Study the drawing (mm; zero at the part's minimum x, y, z) and answer. Coordinates: 2 decimals unless noted, no trailing zeros. Order: outer loops, then holes, each group sorted by start corner. A loop starts at its lowest first (then second) coordinate and runs counter-clockwise, first axis right, second up. Notation, with made-up numbers: M -4,83.5 L 9,83.5 A26 cw 9,100.5 Z; hole C -9,55 d9. An arc over 180 degrees is marked long. One line per item, written item: value. Start each with the question number.
Q1. Straight lines are drawn through the part: line 1 along Z through (x, y) = (4.88, 5.5) (1 decimal); line 2 along Z through (x, y) = (28.73, 6.95); line 3 along Y through (x, z) = (31.5, 18). For each, find the intervals that lie inside material, in ascending order. Write a range as [from, to].
Q2. The part is cut by section A-A on y = 2.25. Give the vertices of the cut face in (x, z), then the cut area to 3 significant figures.
Q3. The part is cut by section D-D on x = 28.73. Give the vertices of the cut face in (y, z).
Q4. The part is cut by section B-B on x = 4.88. Give the vertices of the cut face in (y, z) (1 decimal), then the cut area to 3 significant figures.
Q5. The part is cut by section C-C on z = 23. Give the vertices of the cut face in (x, y).
Q6. Each of these flat-tipped pins is pushed along its axis until it touches: pin 1 Ø1.5 at (x, y) = (5.5, 1.5) entering from -Z; pin 2 Ø2.5 at (x, y) = (17, 1.5) entering from +Z; pin 3 Ø5 at (x, z) = (9, 13.5) entering from -Y; pin 4 Ø4 at (x, z) = (23, 24) entering from -Y. Where does it stop, or does it pass through?
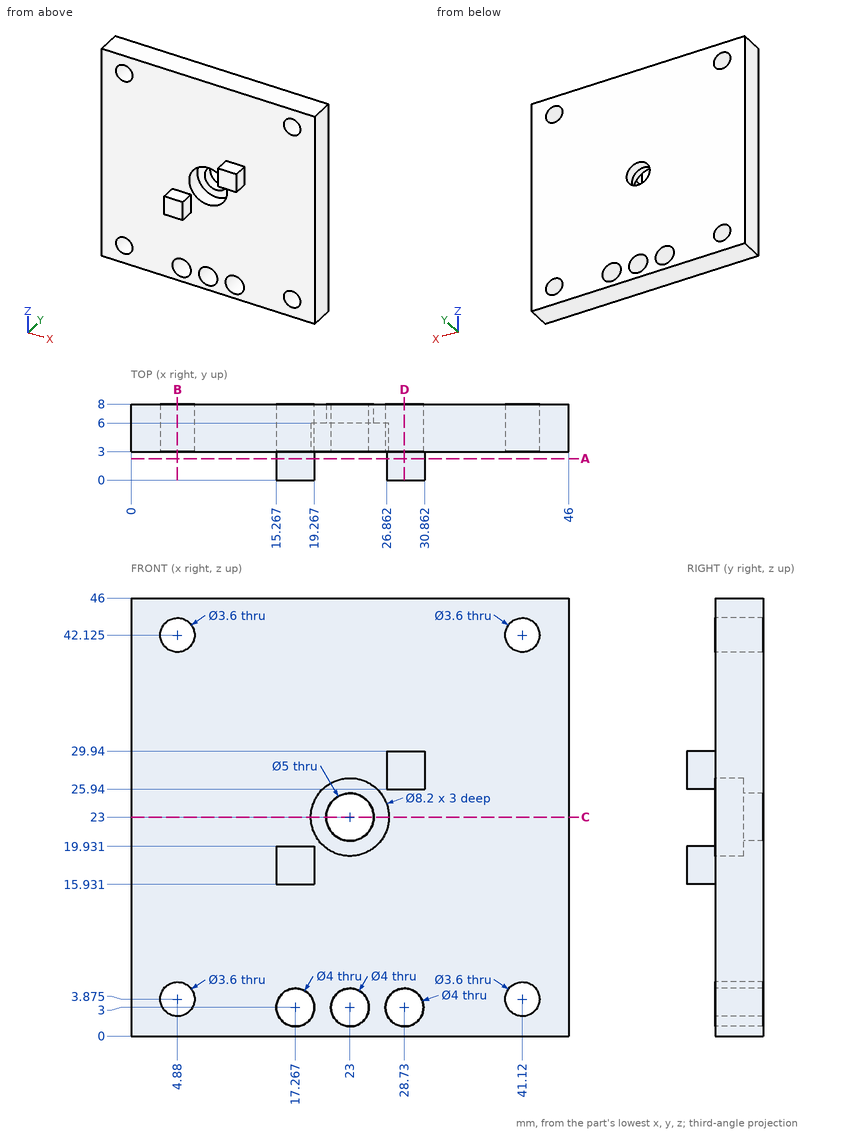
Output:
1. line 1: z = [0, 2.1], [5.7, 40.3], [43.9, 46]
1. line 2: z = [0, 1], [5, 46]
1. line 3: y = [3, 8]
2. outline: M 15.27,15.93 L 19.27,15.93 L 19.27,19.93 L 15.27,19.93 Z; M 26.86,25.94 L 30.86,25.94 L 30.86,29.94 L 26.86,29.94 Z
2. area: 32.0 mm^2
3. outline: M 0,25.94 L 3,25.94 L 3,5 L 8,5 L 8,46 L 3,46 L 3,29.94 L 0,29.94 Z; M 3,0 L 8,0 L 8,1 L 3,1 Z
4. outline: M 3,0 L 8,0 L 8,2.1 L 3,2.1 Z; M 3,5.7 L 8,5.7 L 8,40.3 L 3,40.3 Z; M 3,43.9 L 8,43.9 L 8,46 L 3,46 Z
4. area: 194 mm^2
5. outline: M 0,3 L 18.9,3 L 18.9,6 L 20.5,6 L 20.5,8 L 0,8 Z; M 25.5,6 L 27.1,6 L 27.1,3 L 46,3 L 46,8 L 25.5,8 Z
6. pin 1: passes through
6. pin 2: stops at z = 19.93
6. pin 3: stops at y = 3
6. pin 4: stops at y = 6
